Source: CAD feature listing. Evaluate the final solid. Frame: model axes, mm. Face numbers are marked on the shaded views. A direction names the side the tool comes from. Give positions to 0.01 mm unless a question says otherwise; leave off trailing zeros. Order: outer loops, then holes, each group sorted by start corner. A loop starts at its lowest first (then second) coordinate and runs counter-clockwise, first axis right, second up. Notation, with made-up numbers: M 30,62.5 L 62,62.5 A37 cw 62,101.5 Z; hole C 80,-27.5 d2. An arc over 180 degrees is marked long. Answer in a Markdown table with one row per item. Add a question column.
(1) Mould query, pull axis X, two halves, no side actions, for the marked faces 1, 2, 3 and 4. Classes: pulls with the +X half, pulls with the -X half, needs draft (parallel to the pull), parting line crosses it, or undercut.
(2) Section query B-B, the plane x = 45.5. Return loops of the section in (y, z).
(3) Pin query (flat end, axial travel): P1, Ø2.5, axis at x = 22, z = -39, coming from the +Y side; P2, Ø5.5, axis at x = 71.5, y = 33.5, coming from the +Z side; P3, Ø8, axis at x = 45, z = -41, coming from the +Y side. Return the tip coordinate at first contact, or that it passes through.
(4) Section query A-A, the plane z = 4.5. Return loops of the section in (x, y), plus the area to 3 significant figures.
(5) Section query C-C, the plane y = 37. Count the separate pieces of the cut face and the enclosed holes in it, plus the area to 3 significant figures.
(6) Set-up query: the marked faces 5 and 6. Return all of +Z, -Z, +X, -X, +Y, -Y with unobstructed straight access to the full face (end or side cutting, diameter ignored); none if empty.
(7) Material intervals for line 1 along X through (y, z) = (15.5, -23); line 2 along Z through (x, y) = (-57, 15.5); line 3 along Z through (x, y) = (-81.5, 38.7), sorted ascending.
from build123d import *
from build123d.topology import SkipClean

# Parameters (mm, degrees)
SKETCH1_W           = 150
SKETCH1_H           = 110
BOSS_EXTRUDE1_DEPTH = 40
SHELL1_T            = -5
SKETCH2_R           = 6
SKETCH2_R_2         = 2.25
BOSS_EXTRUDE2_DEPTH = 7.5
SKETCH3_W           = 100
SKETCH3_H           = 100
BOSS_EXTRUDE3_DEPTH = 8
SKETCH4_W           = 99
SKETCH4_H           = 99
CUT_EXTRUDE1_DEPTH  = 8
SKETCH6_R           = 4
SKETCH6_R_2         = 1.5
BOSS_EXTRUDE4_DEPTH = 3
SKETCH7_R           = 1.5
CUT_EXTRUDE2_DEPTH  = 117.496977326
FILLET1_R           = 5
FILLET2_R           = 1.5
SKETCH8_R           = 2.25
BOSS_EXTRUDE5_DEPTH = 5
BOSS_EXTRUDE6_START = 8
BOSS_EXTRUDE6_DEPTH = 8
SKETCH10_R          = 2
CUT_EXTRUDE3_DEPTH  = 10
BOSS_EXTRUDE7_START = 8
SKETCH11_W          = 99
SKETCH11_H          = 99
SKETCH11_R          = 1.5
BOSS_EXTRUDE7_DEPTH = 8
SKETCH12_R          = 2.25
BOSS_EXTRUDE8_DEPTH = 35
CUT_EXTRUDE4_DEPTH  = 40
CUT_EXTRUDE5_DEPTH  = 130


with BuildPart() as part:
    # Sketch1 → Boss-Extrude1 (new body)
    with BuildSketch(Plane(origin=(0, 0, 0), x_dir=(1, 0, 0), z_dir=(0, 1, 0))):
        Rectangle(SKETCH1_W, SKETCH1_H)
    extrude(amount=BOSS_EXTRUDE1_DEPTH)

    # Shell1
    shell1_openings = [part.faces().sort_by_distance(p)[0] for p in [
        (0, 40, 0),
    ]]
    offset(amount=SHELL1_T, openings=shell1_openings, kind=Kind.INTERSECTION)

    # Sketch2 → Boss-Extrude2 (add)
    # profile 1 of 4: a face of its own
    with BuildSketch(Plane.XZ):
        with Locations((84.450112608, -28.114678388)):
            Circle(SKETCH2_R)
        with Locations(Location((84.450112608, -28.114678388, 0), (0, 0, 270))):
            Circle(SKETCH2_R_2, mode=Mode.SUBTRACT)
    # profile 2 of 4: a face of its own
    with BuildSketch(Plane.XZ):
        with BuildLine():
            ThreePointArc((84.450112608, -34.114678388), (78.450112608, -28.114678388), (84.450112608, -22.114678388))
            Line((84.450112608, -22.114678388), (75, -22.114678388))
            Line((75, -22.114678388), (75, -34.114678388))
            Line((75, -34.114678388), (84.450112608, -34.114678388))
        make_face()
    # profile 3 of 4: a face of its own
    with BuildSketch(Plane.XZ):
        with Locations((-62.149887392, 63.385321612)):
            Circle(SKETCH2_R)
        with Locations(Location((-62.149887392, 63.385321612, 0), (0, 0, 270))):
            Circle(SKETCH2_R_2, mode=Mode.SUBTRACT)
    # profile 4 of 4: a face of its own
    with BuildSketch(Plane.XZ):
        with BuildLine():
            Line((-68.149887392, 55), (-56.149887392, 55))
            Line((-56.149887392, 55), (-56.149887392, 63.385321612))
            ThreePointArc((-56.149887392, 63.385321612), (-62.149887392, 57.385321612), (-68.149887392, 63.385321612))
            Line((-68.149887392, 63.385321612), (-68.149887392, 55))
        make_face()
    extrude(amount=-BOSS_EXTRUDE2_DEPTH)

    # Sketch3 → Boss-Extrude3 (add)
    with BuildSketch(Plane(origin=(0, 5, 0), x_dir=(1, 0, 0), z_dir=(0, 1, 0))):
        with Locations((-20, 0)):
            Rectangle(SKETCH3_W, SKETCH3_H)
    extrude(amount=BOSS_EXTRUDE3_DEPTH)

    # Sketch4 → Cut-Extrude1 (cut)
    with BuildSketch(Plane.XZ):
        with Locations((-20, 0)):
            Rectangle(SKETCH4_W, SKETCH4_H)
    extrude(amount=-CUT_EXTRUDE1_DEPTH, mode=Mode.SUBTRACT)

    # Sketch6 → Boss-Extrude4 (add)
    # profile 1 of 4: a face of its own
    with BuildSketch(Plane(origin=(0, 13, 0), x_dir=(1, 0, 0), z_dir=(0, 1, 0))):
        with Locations(Location((21.54565415, 39.178286409, 0), (0, 0, 270))):
            Circle(SKETCH6_R)
        with Locations(Location((21.54565415, 39.178286409, 0), (0, 0, 270))):
            Circle(SKETCH6_R_2, mode=Mode.SUBTRACT)
    # profile 2 of 4: a face of its own
    with BuildSketch(Plane(origin=(0, 13, 0), x_dir=(1, 0, 0), z_dir=(0, 1, 0))):
        with Locations(Location((21.54565415, -35.021713591, 0), (0, 0, 270))):
            Circle(SKETCH6_R)
        with Locations(Location((21.54565415, -35.021713591, 0), (0, 0, 270))):
            Circle(SKETCH6_R_2, mode=Mode.SUBTRACT)
    # profile 3 of 4: a face of its own
    with BuildSketch(Plane(origin=(0, 13, 0), x_dir=(1, 0, 0), z_dir=(0, 1, 0))):
        with Locations(Location((-62.65434585, -35.021713591, 0), (0, 0, 270))):
            Circle(SKETCH6_R)
        with Locations(Location((-62.65434585, -35.021713591, 0), (0, 0, 270))):
            Circle(SKETCH6_R_2, mode=Mode.SUBTRACT)
    # profile 4 of 4: a face of its own
    with BuildSketch(Plane(origin=(0, 13, 0), x_dir=(1, 0, 0), z_dir=(0, 1, 0))):
        with Locations(Location((-62.65434585, 39.178286409, 0), (0, 0, 270))):
            Circle(SKETCH6_R)
        with Locations(Location((-62.65434585, 39.178286409, 0), (0, 0, 270))):
            Circle(SKETCH6_R_2, mode=Mode.SUBTRACT)
    extrude(amount=BOSS_EXTRUDE4_DEPTH)

    # Sketch7 → Cut-Extrude2 (cut, through all)
    with SkipClean():  # the faces are left unmerged after this step: merging them gives an invalid solid
        with BuildSketch(Plane(origin=(0, 16, 0), x_dir=(1, 0, 0), z_dir=(0, 1, 0))):
            with Locations(Location((-62.65434585, -35.021713591, 0), (0, 0, 90))):
                Circle(SKETCH7_R)
            with Locations(Location((-62.65434585, 39.178286409, 0), (0, 0, 90))):
                Circle(SKETCH7_R)
            with Locations(Location((21.54565415, -35.021713591, 0), (0, 0, 90))):
                Circle(SKETCH7_R)
            with Locations(Location((21.54565415, 39.178286409, 0), (0, 0, 90))):
                Circle(SKETCH7_R)
        extrude(amount=-CUT_EXTRUDE2_DEPTH, mode=Mode.SUBTRACT)
    add(part.part.scale(1), mode=Mode.REPLACE)  # the faces are merged on a copy

    # Fillet1
    fillet1_edges = [part.edges().sort_by_distance(p)[0] for p in [
        (70, 22.5, 50),
        (70, 22.5, -50),
        (-70, 26.5, -50),
        (-70, 26.5, 50),
        (75, 3.75, -34.114678388),
        (75, 3.75, -22.114678388),
        (-56.149887392, 3.75, 55),
        (-68.149887392, 3.75, 55),
        (75, 20, 55),
        (-75, 20, -55),
        (75, 20, -55),
    ]]
    fillet(fillet1_edges, radius=FILLET1_R)

    # Fillet2
    fillet2_edges = [part.edges().sort_by_distance(p)[0] for p in [
        (-75, 20, 55),
    ]]
    fillet(fillet2_edges, radius=FILLET2_R)

    # Sketch8 → Boss-Extrude5 (add)
    # profile 1 of 2: a face of its own
    with BuildSketch(Plane(origin=(0, 40, 0), x_dir=(1, 0, 0), z_dir=(0, 1, 0))):
        with BuildLine():
            Line((-75, 40.75), (-81.5, 40.75))
            ThreePointArc((-81.5, 40.75), (-87.25, 35), (-81.5, 29.25))
            Line((-81.5, 29.25), (-75, 29.25))
            Line((-75, 29.25), (-75, 40.75))
        make_face()
        with Locations(Location((-81.5, 35, 0), (0, 0, 270))):
            Circle(SKETCH8_R, mode=Mode.SUBTRACT)
    # profile 2 of 2: a face of its own
    with BuildSketch(Plane(origin=(0, 40, 0), x_dir=(1, 0, 0), z_dir=(0, 1, 0))):
        with BuildLine():
            Line((75, -40.75), (81.5, -40.75))
            ThreePointArc((81.5, -40.75), (87.25, -35), (81.5, -29.25))
            Line((81.5, -29.25), (75, -29.25))
            Line((75, -29.25), (75, -40.75))
        make_face()
        with Locations(Location((81.5, -35, 0), (0, 0, 270))):
            Circle(SKETCH8_R, mode=Mode.SUBTRACT)
    extrude(amount=-BOSS_EXTRUDE5_DEPTH)

    # Sketch9 → Boss-Extrude6 (add)
    with BuildSketch(Plane(origin=(0, 5, 0), x_dir=(1, 0, 0), z_dir=(0, 1, 0)).offset(BOSS_EXTRUDE6_START)):
        with BuildLine():
            Line((30, -50), (65, -50))
            ThreePointArc((65, -50), (68.535533906, -48.535533906), (70, -45))
            Line((70, -45), (70, 45))
            ThreePointArc((70, 45), (68.535533906, 48.535533906), (65, 50))
            Line((65, 50), (30, 50))
            Line((30, 50), (30, -50))
        make_face()
    extrude(amount=-BOSS_EXTRUDE6_DEPTH)

    # Sketch10 → Cut-Extrude3 (cut)
    with BuildSketch(Plane(origin=(75, 0, 0), x_dir=(0, 0, -1), z_dir=(1, 0, 0))):
        with BuildLine():
            Line((7, 40), (7, 30))
            ThreePointArc((7, 30), (9, 32), (11, 30))
            Line((11, 30), (11, 40))
            Line((11, 40), (7, 40))
        make_face()
        with Locations((9, 30)):
            Circle(SKETCH10_R)
        with BuildLine():
            Line((30, 40), (26, 40))
            Line((26, 40), (26, 25))
            ThreePointArc((26, 25), (28, 27), (30, 25))
            Line((30, 25), (30, 40))
        make_face()
        with Locations((28, 25)):
            Circle(SKETCH10_R)
    extrude(amount=-CUT_EXTRUDE3_DEPTH, mode=Mode.SUBTRACT)

    # Sketch11 → Boss-Extrude7 (add)
    with BuildSketch(Plane.XZ.offset(-8).offset(BOSS_EXTRUDE7_START)):
        with Locations((-20, 0)):
            Rectangle(SKETCH11_W, SKETCH11_H)
        with Locations(Location((21.54565415, 35.021713591, 0), (0, 0, 270))):
            Circle(SKETCH11_R, mode=Mode.SUBTRACT)
        with Locations(Location((-62.65434585, 35.021713591, 0), (0, 0, 270))):
            Circle(SKETCH11_R, mode=Mode.SUBTRACT)
        with Locations(Location((21.54565415, -39.178286409, 0), (0, 0, 270))):
            Circle(SKETCH11_R, mode=Mode.SUBTRACT)
        with Locations(Location((-62.65434585, -39.178286409, 0), (0, 0, 270))):
            Circle(SKETCH11_R, mode=Mode.SUBTRACT)
    extrude(amount=-BOSS_EXTRUDE7_DEPTH)

    # Sketch12 → Boss-Extrude8 (add)
    # profile 1 of 2: a face of its own
    with SkipClean():  # the faces are left unmerged after this step: merging them gives an invalid solid
        with BuildSketch(Plane.XZ.offset(-35)):
            with BuildLine():
                ThreePointArc((-81.5, -29.25), (-87.25, -35), (-81.5, -40.75))
                Line((-81.5, -40.75), (-75, -40.75))
                Line((-75, -40.75), (-75, -29.25))
                Line((-75, -29.25), (-81.5, -29.25))
            make_face()
            with Locations((-81.5, -35)):
                Circle(SKETCH12_R, mode=Mode.SUBTRACT)
        # profile 2 of 2: a face of its own
        with BuildSketch(Plane.XZ.offset(-35)):
            with BuildLine():
                ThreePointArc((81.5, 29.25), (87.25, 35), (81.5, 40.75))
                Line((81.5, 40.75), (75, 40.75))
                Line((75, 40.75), (75, 29.25))
                Line((75, 29.25), (81.5, 29.25))
            make_face()
        extrude(amount=BOSS_EXTRUDE8_DEPTH)
    add(part.part.scale(1), mode=Mode.REPLACE)  # the faces are merged on a copy

    # Sketch13 → Cut-Extrude4 (cut)
    with BuildSketch(Plane.XY.offset(55)):
        Polygon((87.25, 0), (87.25, 40), (81.5, 21.224489796), (81.5, 0), align=None)
        Polygon((81.5, 0), (81.5, 21.224489796), (75, 0), align=None)
        Polygon((-75, 0), (-81.5, 21.224489796), (-81.5, 0), align=None)
        Polygon((-81.5, 21.224489796), (-87.25, 40), (-87.25, 0), (-81.5, 0), align=None)
    extrude(amount=-CUT_EXTRUDE4_DEPTH, mode=Mode.SUBTRACT)

    # Sketch14 → Cut-Extrude5 (cut)
    with BuildSketch(Plane.XY.offset(55)):
        Polygon((-81.5, 21.224489796), (-81.5, 0), (-75, 0), align=None)
        Polygon((-87.25, 0), (-81.5, 0), (-81.5, 21.224489796), (-87.25, 40), align=None)
    extrude(amount=-CUT_EXTRUDE5_DEPTH, mode=Mode.SUBTRACT)


solid = part.part
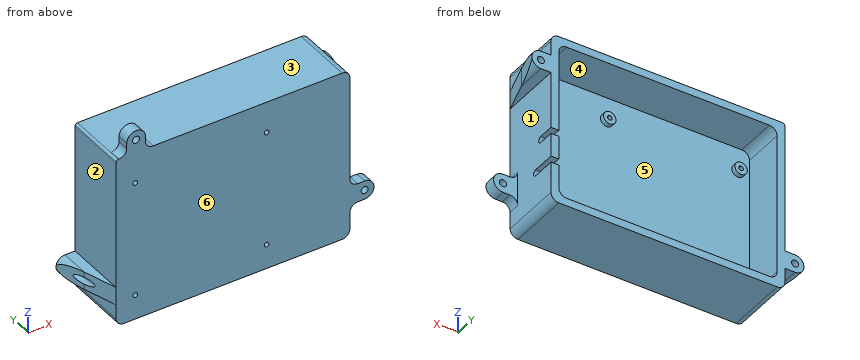
Values follow:
| question | item | result |
|---|---|---|
| 1 | face 1 | pulls with the +X half |
| 1 | face 2 | pulls with the -X half |
| 1 | face 3 | needs draft |
| 1 | face 4 | undercut |
| 2 | outline | M 0,-55 L 40,-55 L 40,-50 L 13,-50 L 13,50 L 40,50 L 40,55 L 0,55 Z |
| 3 | P1 | stops at y = 16 |
| 3 | P2 | stops at z = 55 |
| 3 | P3 | stops at y = 13 |
| 4 | outline | M -75,0 L 75,0 L 75,40 L 70,40 L 70,13 L -70,13 L -70,40 L -75,40 Z |
| 4 | area | 2,220 mm² |
| 5 | separate pieces | 2 |
| 5 | enclosed holes | 2 |
| 5 | area | 2,680 mm² |
| 6 | face 5 | +Y |
| 6 | face 6 | +Z, -Z, +X, -X, -Y |
| 7 | line 1 | x = -75 to -70, 70 to 75 |
| 7 | line 2 | z = -55 to -50, 50 to 55 |
| 7 | line 3 | z = -40.75 to -37.25, -32.75 to -29.25 |
